Check sheet for the modelled part. Datum: model origin and axes. Units: mm. A direction names the side the tool comes from. Give positions to 0.01 mm unless a question says otherwise; leave off trailing zeros. Write each loop counter-clockwise with the first axis right and the second up, starting at its lowest first coordinate (ties: lowest second). Pieces come first, ordered by that corner, then holes. Notation, with made-up numbers: (-8, 46.25) -> (42, 46.25) arc R23 ccw to (42, 69.25) -> close; hole circle Ø8 at (23.5, 3). An arc over 180 degrees is marked (long way). Return JSON: item names as keys, results as strings.
from build123d import *

# Parameters (mm, degrees)
SKETCH1_R           = 6
BOSS_EXTRUDE1_DEPTH = 20
CUT_EXTRUDE1_DEPTH  = 15
BOSS_EXTRUDE2_DEPTH = 75


with BuildPart() as part:
    # Sketch1 → Boss-Extrude1 (new body)
    with BuildSketch(Plane(origin=(0, 0, 0), x_dir=(0, 0, -1), z_dir=(1, 0, 0))):
        Circle(SKETCH1_R)
    extrude(amount=BOSS_EXTRUDE1_DEPTH)

    # Sketch2 → Cut-Extrude1 (cut)
    with BuildSketch(Plane.ZY):
        with BuildLine():
            Line((-2.683281573, 3.1), (2.683281573, 3.1))
            ThreePointArc((2.683281573, 3.1), (4.1, 0), (2.683281573, -3.1))
            Line((2.683281573, -3.1), (-2.683281573, -3.1))
            ThreePointArc((-2.683281573, -3.1), (-4.1, 0), (-2.683281573, 3.1))
        make_face()
    extrude(amount=-CUT_EXTRUDE1_DEPTH, mode=Mode.SUBTRACT)

    # Sketch3 → Boss-Extrude2 (add)
    with BuildSketch(Plane(origin=(20, 0, 0), x_dir=(0, 0, -1), z_dir=(1, 0, 0))):
        with BuildLine():
            Line((2.645751311, 3), (-2.645751311, 3))
            ThreePointArc((-2.645751311, 3), (0, -4), (2.645751311, 3))
        make_face()
    extrude(amount=BOSS_EXTRUDE2_DEPTH)


solid = part.part
(1) Release check for a two-part mould opening along Y. For faces 4 (the flat face through (7, -3.1, 0)), 5 (the cylindrical face through (10, 0, 6)), 6 (the flat face through (57, 3, 0)), 7 (the cylindrical face through (7.4, 0, 4.1)) record: pulls with the +Y half, pulls with the -Y half, needs draft (parallel to the pull), parting line crosses it, or undercut.
Reply:
{"face 4": "undercut", "face 5": "parting line crosses it", "face 6": "pulls with the +Y half", "face 7": "undercut"}
(2) Cross-section at B-B on y = 0. Enter the section's corners in (x, z).
Reply:
{"outline": "(0, -6) -> (20, -6) -> (20, -4) -> (95, -4) -> (95, 4) -> (20, 4) -> (20, 6) -> (0, 6) -> (0, 4.1) -> (15, 4.1) -> (15, -4.1) -> (0, -4.1) -> close"}
(3) Cross-section at D-D on z = 5. Enter the section's corners in (x, y).
Reply:
{"outline": "(0, -3.32) -> (20, -3.32) -> (20, 3.32) -> (0, 3.32) -> close"}
(4) Set-up check for faces 1 (the cylindrical face through (57, -4, 0)), 2 (the cylindrical face through (7.4, 0, -4.1)), 3 (the flat face through (95, 0, 0)): record each of +Z, -Z, +X, -X, +Y, -Y from which the full face is reachable in a straight line by a thin tool's end or side.
Reply:
{"face 1": "+X", "face 2": "-X", "face 3": "+Z, -Z, +X, +Y, -Y"}
(5) Thickness scan on L1, parallel to X at y = -0.25, z = 0.75; L2, parallel to X at y = -4.5, z = -1.5; L3, parallel to Z at x = 9.5, y = 1.25. Record the ranges inside material, lowest first.
Reply:
{"L1": "15 to 95", "L2": "0 to 20", "L3": "-5.87 to -3.9, 3.9 to 5.87"}
(6) Cross-section at A-A on z = 0. Enter the section's corners in (x, y).
Reply:
{"outline": "(0, -6) -> (20, -6) -> (20, -4) -> (95, -4) -> (95, 3) -> (20, 3) -> (20, 6) -> (0, 6) -> (0, 3.1) -> (15, 3.1) -> (15, -3.1) -> (0, -3.1) -> close"}
(7) Depth check by flat-ended pin: pin 1 Ø6 at (x, y) = (59, 1) entering from +Z; pin 2 Ø1.9 at (y, z) = (-1, 0) entering from -X; pin 3 Ø1 at (x, y) = (35.5, -1.5) entering from -Z. Enter the tip coordinate at first touch or a pass-through.
Reply:
{"pin 1": "z = 4", "pin 2": "x = 15", "pin 3": "z = -3.87"}
(8) Cross-section at C-C on x = 73. Enter the section's corners in (y, z), then the cut area to 3 significant figures.
Reply:
{"outline": "(3, -2.65) -> (3, 2.65) arc R4 ccw (long way) to start", "area": "46.6 mm^2"}
